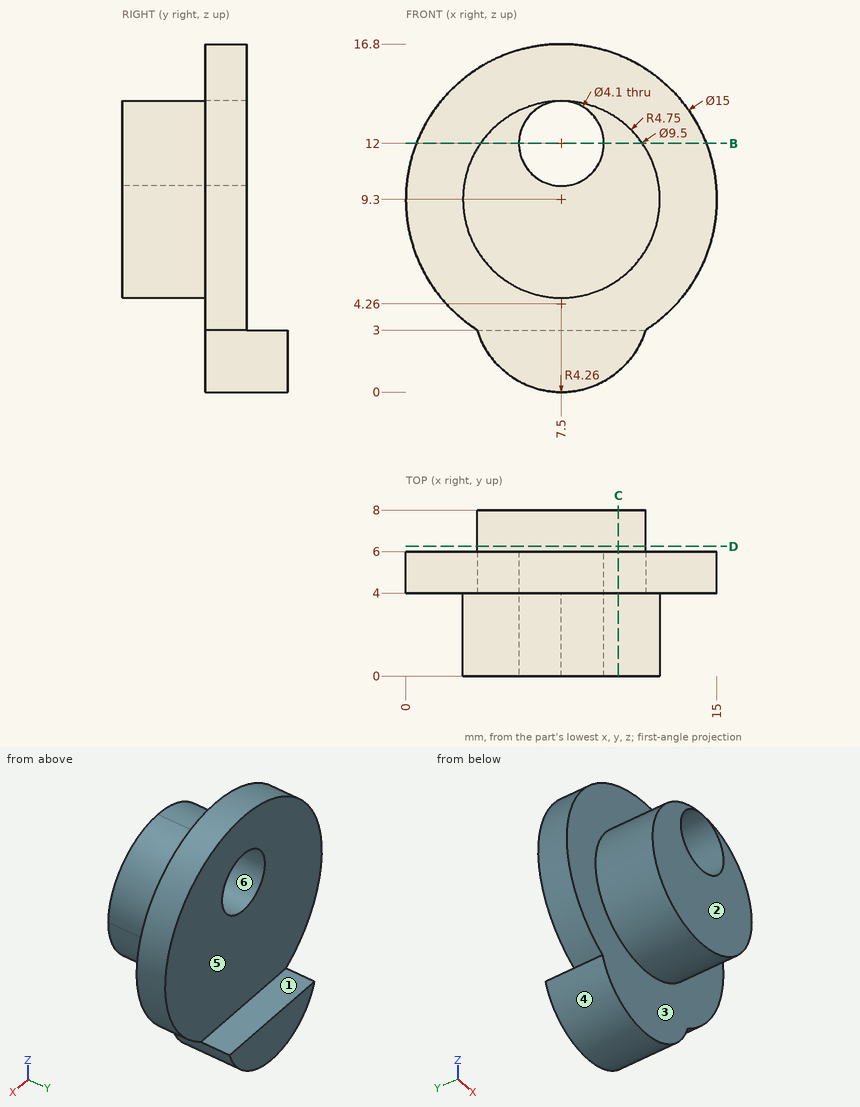
Can you work these out from the drawing? Everything is in mm from the part's minimum corner. A direction names the side the tool comes from. Round coordinates to 2 decimals unless told otherwise and drop trailing zeros. Write each loop counter-clockwise with the first axis right and the second up, starting at its lowest first coordinate (ties: lowest second). Pieces come first, ordered by that corner, then holes. Notation, with made-up numbers: M 38,78 L 76,78 A15 cw 76,102 Z; hole C -6.5,52 d2. An arc over 180 degrees is marked long. Use a Markdown table: item, result.
Item 1: We'd pull the mould along X, two halves only. Please class the marked faces 4, 5 and 6: released by +X, released by -X, zero draft, split by the parting line, or undercut.
Found:
| item | result |
|---|---|
| face 4 | split by the parting line |
| face 5 | zero draft |
| face 6 | undercut |
Item 2: I want a section at B-B (z = 12). List the corners of the cut face in (x, y) for me, and give its area (3 significant figures).
Found:
| item | result |
|---|---|
| outline | M 0.5,4 L 3.59,4 L 3.59,0 L 5.45,0 L 5.45,6 L 0.5,6 Z; M 9.55,0 L 11.41,0 L 11.41,4 L 14.5,4 L 14.5,6 L 9.55,6 Z |
| area | 34.7 mm2 |
Item 3: I want a section at C-C (x = 10.25). List the corners of the cut face in (y, z) for me.
Found:
| item | result |
|---|---|
| outline | M 0,5.43 L 4,5.43 L 4,1.01 L 8,1.01 L 8,3 L 6,3 L 6,16.28 L 4,16.28 L 4,13.17 L 0,13.17 Z |
Item 4: If I drill on line 1 along Z through (x, y) = (7.5, 4.85); line 2 along Y through (x, z) = (10.25, 3.25); line 3 along Y through (x, z) = (11.75, 11), over which ranges is the centre line in solid material (lowest first)? Write a range as [from, to].
Found:
| item | result |
|---|---|
| line 1 | z = [0, 9.95], [14.05, 16.8] |
| line 2 | y = [4, 6] |
| line 3 | y = [0, 6] |
Item 5: I want a section at D-D (y = 6.25). List the corners of the cut face in (x, z) for me, and give its area (3 significant figures).
Found:
| item | result |
|---|---|
| outline | M 3.43,3 A4.26 ccw 11.57,3 Z |
| area | 17.9 mm2 |
Item 6: Which directions (+Z, -Z, +X, -X, +Y, -Y) give clear straight access to the entire face, cutting with the end or side of a thin tool? Please do the marked faces 1, 2 and 3.
Found:
| item | result |
|---|---|
| face 1 | +Z, +X, -X, +Y |
| face 2 | +Z, -Z, +X, -X, -Y |
| face 3 | -Y |
Item 7: For pin 1 Ø0.6 at (x, y) = (6.5, 6.5) entering from +Z; pin 2 Ø6 at (x, z) = (2.5, 14.5) entering from +Y; pin 3 Ø3 at (y, z) = (1.5, 8) entering from -X, each with a flat end and sliding along its axis, tell me the tip position at first contact or that it passes through.
Found:
| item | result |
|---|---|
| pin 1 | stops at z = 3 |
| pin 2 | stops at y = 6 |
| pin 3 | stops at x = 2.75 |
